For this review, take the finished solid that the model builds, in its own axes (mm). A direction names the side the tool comes from. Coordinates: 2 decimals unless noted, no trailing zeros. Write each loop counter-clockwise with the first axis right and the second up, starting at its lowest first coordinate (ties: lowest second). Pieces come first, ordered by that corner, then holes. Notation, with made-up numbers: M 0.25,54.25 L 16.25,54.25 A23 cw 16.25,80.25 Z; hole C 77,14.5 d4. An arc over 180 degrees is marked long. Return JSON: item names as keys, results as strings.
```python
from build123d import *

# Parameters (mm, degrees)
SKETCH_1_W               = 42
SKETCH_1_H               = 42
EXTRUDE_1_DEPTH          = 26
SKETCH_2_W               = 16
SKETCH_2_H               = 4
EXTRUDE_2_DEPTH          = 3.15
CUT_EXTRUDE_1_REACH      = 43.737
CUT_EXTRUDE_START        = -8.5
CUT_EXTRUDE_2_DEPTH      = 10
FILLET_2_R               = 1.5
FILLET_3_R               = 2
SKETCH_10_R              = 11.8
CUT_EXTRUDE_5_DEPTH      = 0.2
SKETCH_11_R              = 11
SKETCH_11_R_2            = 3.65
EXTRUDE_7_DEPTH          = 2.2
SKETCH_12_R              = 3.65
SKETCH_12_R_2            = 2.5
EXTRUDE_8_DEPTH          = 0.3
FILLET_4_R               = 0.3
SKETCH_13_R              = 2.5
EXTRUDE_9_DEPTH          = 17.2
CUT_EXTRUDE_6_DEPTH      = 54.990739947
CUT_EXTRUDE_6_DEPTH_BACK = 14
SKETCH_15_R              = 1.2645
CUT_EXTRUDE_7_DEPTH      = 4.4
CHAMFER_4_SIZE           = 0.3
CHAMFER_5_SIZE           = 0.3
FILLET_5_R               = 0.5


with BuildPart() as part:
    # 草图1 → 凸台-拉伸1 (new body)
    with BuildSketch(Plane.XY):
        Rectangle(SKETCH_1_W, SKETCH_1_H)
    extrude(amount=EXTRUDE_1_DEPTH)

    # 草图2 → 凸台-拉伸2 (add)
    with BuildSketch(Plane(origin=(0, 0, 0), x_dir=(-1, 0, 0), z_dir=(0, 0, -1))):
        with Locations((0, 23)):
            Rectangle(SKETCH_2_W, SKETCH_2_H)
    extrude(amount=-EXTRUDE_2_DEPTH)

    # 草图3 → 切除-拉伸1 (cut, up to next)
    with BuildSketch(Plane(origin=(0, 0, 0), x_dir=(-1, 0, 0), z_dir=(0, 0, -1)), mode=Mode.PRIVATE) as cut_extrude_1_sk1:
        Polygon((-17.075, 21), (-21, 17.075), (-21, 21), align=None)
    cut_extrude_1_tool1 = extrude(cut_extrude_1_sk1.sketch, amount=-CUT_EXTRUDE_1_REACH, mode=Mode.PRIVATE) & part.part
    # 草图3 → 切除-拉伸1 (cut, up to next)
    with BuildSketch(Plane(origin=(0, 0, 0), x_dir=(-1, 0, 0), z_dir=(0, 0, -1)), mode=Mode.PRIVATE) as cut_extrude_1_sk2:
        Polygon((17.075, 21), (21, 17.075), (21, 21), align=None)
    cut_extrude_1_tool2 = extrude(cut_extrude_1_sk2.sketch, amount=-CUT_EXTRUDE_1_REACH, mode=Mode.PRIVATE) & part.part
    # 草图3 → 切除-拉伸1 (cut, up to next)
    with BuildSketch(Plane(origin=(0, 0, 0), x_dir=(-1, 0, 0), z_dir=(0, 0, -1)), mode=Mode.PRIVATE) as cut_extrude_1_sk3:
        Polygon((21, -17.075), (17.075, -21), (21, -21), align=None)
    cut_extrude_1_tool3 = extrude(cut_extrude_1_sk3.sketch, amount=-CUT_EXTRUDE_1_REACH, mode=Mode.PRIVATE) & part.part
    # 草图3 → 切除-拉伸1 (cut, up to next)
    with BuildSketch(Plane(origin=(0, 0, 0), x_dir=(-1, 0, 0), z_dir=(0, 0, -1)), mode=Mode.PRIVATE) as cut_extrude_1_sk4:
        Polygon((-21, -17.075), (-17.075, -21), (-21, -21), align=None)
    cut_extrude_1_tool4 = extrude(cut_extrude_1_sk4.sketch, amount=-CUT_EXTRUDE_1_REACH, mode=Mode.PRIVATE) & part.part
    add(cut_extrude_1_tool1.solids().sort_by_distance((19.691667, 19.691667, 0))[0], mode=Mode.SUBTRACT)
    add(cut_extrude_1_tool2.solids().sort_by_distance((-19.691667, 19.691667, 0))[0], mode=Mode.SUBTRACT)
    add(cut_extrude_1_tool3.solids().sort_by_distance((-19.691667, -19.691667, 0))[0], mode=Mode.SUBTRACT)
    add(cut_extrude_1_tool4.solids().sort_by_distance((19.691667, -19.691667, 0))[0], mode=Mode.SUBTRACT)

    # 草图4 → 切除-拉伸2 (cut)
    with BuildSketch(Plane(origin=(0, 0, 0), x_dir=(-1, 0, 0), z_dir=(0, 0, -1)).offset(CUT_EXTRUDE_START)):
        Polygon((-21, 14.532), (-14.532, 21), (-21, 21), align=None)
        Polygon((14.532, 21), (21, 14.532), (21, 21), align=None)
        Polygon((21, -14.532), (14.532, -21), (21, -21), align=None)
        Polygon((-14.532, -21), (-21, -14.532), (-21, -21), align=None)
    extrude(amount=-CUT_EXTRUDE_2_DEPTH, mode=Mode.SUBTRACT)

    # 圆角2
    fillet_2_edges = [part.edges().sort_by_distance(p)[0] for p in [
        (21, -17.075, 22.25),
        (17.075, -21, 22.25),
        (-21, -17.075, 22.25),
        (-17.075, -21, 22.25),
        (-17.075, 21, 22.25),
        (-21, 17.075, 22.25),
        (17.075, 21, 22.25),
        (21, 17.075, 22.25),
        (17.075, -21, 4.25),
        (21, -17.075, 4.25),
        (-21, -17.075, 4.25),
        (-17.075, -21, 4.25),
        (-17.075, 21, 4.25),
        (-21, 17.075, 4.25),
        (21, 17.075, 4.25),
        (17.075, 21, 4.25),
    ]]
    fillet(fillet_2_edges, radius=FILLET_2_R)

    # 圆角3
    fillet_3_edges = [part.edges().sort_by_distance(p)[0] for p in [
        (-21, -14.532, 13.5),
        (-14.532, -21, 13.5),
        (-14.532, 21, 13.5),
        (-21, 14.532, 13.5),
        (21, 14.532, 13.5),
        (14.532, 21, 13.5),
        (14.532, -21, 13.5),
        (21, -14.532, 13.5),
    ]]
    fillet(fillet_3_edges, radius=FILLET_3_R)

    # 草图10 → 切除-拉伸5 (cut)
    with BuildSketch(Plane.XY.offset(26)):
        Circle(SKETCH_10_R)
    extrude(amount=-CUT_EXTRUDE_5_DEPTH, mode=Mode.SUBTRACT)

    # 草图11 → 凸台-拉伸7 (add)
    with BuildSketch(Plane.XY.offset(25.8)):
        Circle(SKETCH_11_R)
        Circle(SKETCH_11_R_2, mode=Mode.SUBTRACT)
    extrude(amount=EXTRUDE_7_DEPTH)

    # 草图12 → 凸台-拉伸8 (add)
    with BuildSketch(Plane.XY.offset(25.8)):
        Circle(SKETCH_12_R)
        Circle(SKETCH_12_R_2, mode=Mode.SUBTRACT)
    extrude(amount=EXTRUDE_8_DEPTH)

    # 圆角4
    fillet_4_edges = [part.edges().sort_by_distance(p)[0] for p in [
        (-2.5, 0, 26.1),
    ]]
    fillet(fillet_4_edges, radius=FILLET_4_R - 0.0001)  # a hair under: the kernel refuses the full size

    # 草图13 → 凸台-拉伸9 (add)
    with BuildSketch(Plane.XY.offset(25.8)):
        with Locations(Location((0, 0, 0), (0, 0, 180))):
            Circle(SKETCH_13_R)
    extrude(amount=EXTRUDE_9_DEPTH)

    # 草图14 → 切除-拉伸6 (cut, two sides: drawn at the far end of the back side and taken through both)
    with BuildSketch(Plane.XY.offset(43).offset(-CUT_EXTRUDE_6_DEPTH_BACK)):
        Polygon((-75.850602173, 2), (-1.5, 2), (1.5, 2), (75.850602173, 2), (75.850602173, 150.701204346), (-75.850602173, 150.701204346), align=None)
    extrude(amount=CUT_EXTRUDE_6_DEPTH + CUT_EXTRUDE_6_DEPTH_BACK, mode=Mode.SUBTRACT)

    # 草图15 → 切除-拉伸7 (cut)
    with BuildSketch(Plane.XY.offset(26)):
        with Locations((-15.5, 15.5)):
            Circle(SKETCH_15_R)
        with Locations((15.5, 15.5)):
            Circle(SKETCH_15_R)
        with Locations((15.5, -15.5)):
            Circle(SKETCH_15_R)
        with Locations((-15.5, -15.5)):
            Circle(SKETCH_15_R)
    extrude(amount=-CUT_EXTRUDE_7_DEPTH, mode=Mode.SUBTRACT)

    # 倒角4
    chamfer_4_edges = [part.edges().sort_by_distance(p)[0] for p in [
        (-11, 0, 28),
    ]]
    chamfer(chamfer_4_edges, length=CHAMFER_4_SIZE)

    # 倒角5
    chamfer_5_edges = [part.edges().sort_by_distance(p)[0] for p in [
        (-19.0375, -19.0375, 26),
        (-21, 0, 26),
        (19.0375, -19.0375, 26),
        (21, 0, 26),
        (19.0375, 19.0375, 26),
        (0, 21, 26),
        (-19.0375, 19.0375, 26),
        (0, -21, 26),
        (17.027704805, 20.885819299, 26),
        (20.885819299, 17.027704805, 26),
        (20.885819299, -17.027704805, 26),
        (17.027704805, -20.885819299, 26),
        (-17.027704805, 20.885819299, 26),
        (-20.885819299, 17.027704805, 26),
        (-17.027704805, -20.885819299, 26),
        (-20.885819299, -17.027704805, 26),
    ]]
    chamfer(chamfer_5_edges, length=CHAMFER_5_SIZE)

    # 圆角5
    fillet_5_edges = [part.edges().sort_by_distance(p)[0] for p in [
        (-21, 0, 0),
        (-12.226839828, 21, 0),
        (0, -21, 0),
        (21, 0, 0),
        (19.0375, -19.0375, 0),
        (-19.0375, -19.0375, 0),
        (-19.0375, 19.0375, 0),
        (12.226839828, 21, 0),
        (19.0375, 19.0375, 0),
        (17.027704805, 20.885819299, 0),
        (20.885819299, 17.027704805, 0),
        (20.885819299, -17.027704805, 0),
        (17.027704805, -20.885819299, 0),
        (-20.885819299, 17.027704805, 0),
        (-17.027704805, 20.885819299, 0),
        (-20.885819299, -17.027704805, 0),
        (-17.027704805, -20.885819299, 0),
        (-8, 23, 0),
        (0, 25, 0),
        (8, 23, 0),
    ]]
    fillet(fillet_5_edges, radius=FILLET_5_R)


solid = part.part
```
1. Draft analysis for pull direction Z (two halves, no side actions). For faces 1 (the face through (0, 25, 2)), 2 (the face through (18.915, -18.958, 0.15)), 3 (the face through (-18, 18, 18.5)), state which applies: +Z half, -Z half, draft (parallel to the pull), parting line (faces both ways), or undercut.
Checks:
{"face 1": "draft", "face 2": "-Z half", "face 3": "undercut"}
2. For faces 4 (the face through (20.85, 14.46, 13.57)), 5 (the face through (-17.8, -17.73, 13.43)), 6 (the face through (15, 16, 21.6)), 7 (the face through (-8, 23, 2)), 8 (the face through (20.85, -14.46, 13.57)), list the 3-axis set-ups (+Z, -Z, +X, -X, +Y, -Y) from which the entire face can be reached by the end or side of a thin tool; tool diameter is ignored.
Checks:
{"face 4": "+X, +Y", "face 5": "-X, -Y", "face 6": "+Z", "face 7": "+Z, -Z, -X, +Y", "face 8": "+X, -Y"}
3. Clearance check with flat-ended pins moving along their axes: pin 1 Ø2 at (x, y) = (-18, 18.5) entering from +Z; pin 2 Ø2 at (x, y) = (-15.5, 15.5) entering from +Z; pin 3 Ø3 at (x, y) = (-6, -1) entering from +Z. State where each tip first meets the part, or that it passes through.
Checks:
{"pin 1": "z = 26", "pin 2": "z = 21.6", "pin 3": "z = 28"}
4. We need section C-C (z = 13). State the section outline as (x, y) points.
Checks:
{"outline": "M -21,-13.7 A2 ccw -20.41,-15.12 L -15.12,-20.41 A2 ccw -13.7,-21 L 13.7,-21 A2 ccw 15.12,-20.41 L 20.41,-15.12 A2 ccw 21,-13.7 L 21,13.7 A2 ccw 20.41,15.12 L 15.12,20.41 A2 ccw 13.7,21 L -13.7,21 A2 ccw -15.12,20.41 L -20.41,15.12 A2 ccw -21,13.7 Z"}
5. We need section B-B (z = 20). State the section outline as (x, y) points, plus the area to 3 significant figures.
Checks:
{"outline": "M -21,-16.45 A1.5 ccw -20.56,-17.51 L -17.51,-20.56 A1.5 ccw -16.45,-21 L 16.45,-21 A1.5 ccw 17.51,-20.56 L 20.56,-17.51 A1.5 ccw 21,-16.45 L 21,16.45 A1.5 ccw 20.56,17.51 L 17.51,20.56 A1.5 ccw 16.45,21 L -16.45,21 A1.5 ccw -17.51,20.56 L -20.56,17.51 A1.5 ccw -21,16.45 Z", "area": "1,730 mm2"}
6. Wall thickness on L1, parallel to Y at x = 0, z = 26.7; L2, parallel to Y at x = 15.5, z = 25; L3, parallel to Z at x = -16.5, y = 11: over which ranges is each line inside the solid? List them lowest first. Write a range as from..to.
Checks:
{"L1": "-11..-3.65, -2.5..2.5, 3.65..11", "L2": "-21..-16.76, -14.24..14.24, 16.76..21", "L3": "0..26"}
